The model under review builds one solid part; all positions refer to its coordinate system, in mm. A direction names the side the tool comes from. Coordinates: 2 decimals unless noted, no trailing zeros. Loops run counter-clockwise (first coordinate to the right, second up) from the corner with the lowest first, then second, coordinate; pieces in that order, holes last. Notation, with made-up numbers: M -39,-13.75 L 16,-13.75 A20 cw 16,-2.75 Z; hole C 59.5,-18 d3. An arc over 180 degrees is marked long. Use one line per item in the form item = value.
```python
from build123d import *

# Parameters (mm, degrees)
FILLET1_R          = 2.54
SKETCH2_R          = 3.175
CUT_EXTRUDE1_DEPTH = 19.238986472
CIRPATTERN1_COUNT  = 4


with BuildPart() as part:
    # Sketch1 → Revolve1 (revolve)
    with BuildSketch(Plane.XY, mode=Mode.PRIVATE) as revolve1_sk:
        Polygon((6.35, 0), (6.35, 15.875), (4.7625, 15.875), (2.54, 13.318306215), (2.54, 12.810306215), (4.826, 12.810306215), (4.826, 0), align=None)
    revolve(revolve1_sk.sketch.rotate(Axis((0, 0, 0), (0, 1, 0)), 90), axis=Axis((0, 0, 0), (0, 1, 0)))

    # Fillet1
    # the kernel refuses this fillet: 2.54 mm, written as the material it takes off along each edge
    with BuildSketch(Plane(origin=(0, 15.875, 0), x_dir=(0, 0, -1), z_dir=(1, 0, 0))) as fillet1_piece_1:
        with BuildLine():
            CenterArc((3.81, -2.35464302), FILLET1_R, 0, 67.975687163)
            Line((4.7625, 0), (4.78155, 0.04709286))
            ThreePointArc((4.78155, 0.04709286), (5.55625, 0.0508), (6.35, 0.0508))
            Line((6.35, 0.0508), (6.4008, 0))
            Line((6.4008, 0), (6.4008, -2.35464302))
            Line((6.4008, -2.35464302), (6.35, -2.35464302))
        make_face()
    revolve(axis=Axis((0, 15.875, 0), (0, 1, 0)), mode=Mode.SUBTRACT)

    # Sketch2 → Cut-Extrude1 (cut, symmetric)
    with BuildSketch(Plane(origin=(0, 0, 0), x_dir=(0, 0, -1), z_dir=(1, 0, 0))):
        with Locations((0, 6.985)):
            Circle(SKETCH2_R)
    cut_extrude1 = extrude(amount=CUT_EXTRUDE1_DEPTH, both=True, mode=Mode.SUBTRACT)

    # CirPattern1: Cut-Extrude1 ×4 about axis
    cirpattern1_axis = Axis((0, 12.810306215, 0), (0, -1, 0))
    for i in range(1, CIRPATTERN1_COUNT):
        add(cut_extrude1.rotate(cirpattern1_axis, i * 360 / CIRPATTERN1_COUNT), mode=Mode.SUBTRACT)


solid = part.part
```
1. The part is to be moulded in two halves that separate along Y. For faces 3 (the face through (-2.52, 13.06, 0.33)), 4 (the face through (-2.625, 13.442, 0.345)), 5 (the face through (2, 12.81, 2)), 6 (the face through (1.71, 9.66, -4.97)), say which applies: pulls with the +Y half, pulls with the -Y half, needs draft (parallel to the pull), parting line crosses it, or undercut.
Response values:
face_3 = needs draft
face_4 = pulls with the +Y half
face_5 = pulls with the -Y half
face_6 = undercut
2. Add section D-D (y = 2.5). State the section outline as (x, z) points.
Response values:
outline = C 0,0 d12.7; hole C 0,0 d9.65
3. Add section C-C (y = 4.5). State the section outline as (x, z) points, then the cut area to 3 significant figures.
Response values:
outline = M -6.03,-1.98 A6.35 ccw -1.98,-6.03 L -1.98,-4.4 A4.83 cw -4.4,-1.98 Z; M -6.03,1.98 L -4.4,1.98 A4.83 cw -1.98,4.4 L -1.98,6.03 A6.35 ccw Z; M 1.98,-6.03 A6.35 ccw 6.03,-1.98 L 4.4,-1.98 A4.83 cw 1.98,-4.4 Z; M 1.98,4.4 A4.83 cw 4.4,1.98 L 6.03,1.98 A6.35 ccw 1.98,6.03 Z
area = 28.9 mm^2
4. Add section A-A (x = 0). Count the separate pieces of the cut face and the enclosed holes in it, then the cut area to 3 significant figures.
Response values:
separate_pieces = 4
enclosed_holes = 0
area = 35.3 mm^2
5. Insertion check: P1, Ø3, axis at y = 8.5, z = -4, coming from the -X side; P2, Ø1.5, axis at y = 6.5, z = -2.5, coming from the +X side; P3, Ø4, axis at y = 11, z = -5, coming from the -X side. Each pin has a flat end and moves straight along its axis. Give the tip position at first contact, or say it passes through.
Response values:
P1 = -5.82
P2 = 5.6
P3 = -5.6
6. Machinability: for faces 1 (the face through (5.01, 7.94, -3.03)), 2 (the face through (-3.26, 6.32, 3.56)), which of the approach directions +Z, -Z, +X, -X, +Y, -Y give a long, thin tool a straight path to every point of the face, cutting with its end or side? Answer none if there is none.
Response values:
face_1 = +X, -X
face_2 = -Y
7. Wall thickness on line 1 along Y through (x, z) = (0.25, -5.25); line 2 along Z through (x, y) = (0.25, 11); line 3 along X through (y, z) = (5.5, 5.5): over which ranges is each line inside the solid? List them lowest first. Write a range as from..to.
Response values:
line_1 = 0..3.82, 10.15..15.61
line_2 = -6.35..-4.82, 4.82..6.35
line_3 = -3.17..-2.81, 2.81..3.17
